```python
from build123d import *

# Parameters (mm, degrees)
F0_R     = 15
F0_R_2   = 13
F1_DEPTH = 2
F2_DEPTH = 20
F3_R     = 5
F4_SIZE  = 1.4
F5_R     = 1.4


with BuildPart() as f1:
    # F0 (on Top) → F1 (new body)
    with BuildSketch(Plane.XY):
        Circle(F0_R)
        Circle(F0_R_2, mode=Mode.SUBTRACT)
        Circle(F0_R_2)
    extrude(amount=F1_DEPTH)

    # F0 (on Top) → F2 (join)
    with BuildSketch(Plane.XY):
        Circle(F0_R)
        Circle(F0_R_2, mode=Mode.SUBTRACT)
    extrude(amount=F2_DEPTH)

    # F3
    f3_edges = [f1.edges().sort_by_distance(p)[0] for p in [
        (-13, 0, 2),
    ]]
    fillet(f3_edges, radius=F3_R)

    # F4
    f4_edges = [f1.edges().sort_by_distance(p)[0] for p in [
        (-13, 0, 20),
    ]]
    chamfer(f4_edges, length=F4_SIZE)

    # F5
    f5_edges = [f1.edges().sort_by_distance(p)[0] for p in [
        (-15, 0, 0),
    ]]
    fillet(f5_edges, radius=F5_R)


solid = f1.part
```
Geometry: final body of the model. Coordinates: model frame, mm. A direction names the side the tool comes from. Coordinates: 2 decimals unless noted, no trailing zeros. Loops run counter-clockwise (first coordinate to the right, second up) from the corner with the lowest first, then second, coordinate; pieces in that order, holes last. Notation, with made-up numbers: (10, 53) -> (35, 53) arc R21 cw to (35, 74) -> close; hole circle Ø7 at (35, -23.75). An arc over 180 degrees is marked (long way). Use a Markdown table: item, result. Add a question column.
(1) Section query A-A, the plane y = 0. Return loops of the section in (x, z).
(2) Mould query, pull axis Y, two halves, no side actions, for faces 3 (the cylindrical face through (-14.985, 0.66, 10.57)), 4 (the cylindrical face through (-10.316, -7.91, 12.719)), 5 (the flat face through (0, 0, 0)). Classes: pulls with the +Y half, pulls with the -Y half, needs draft (parallel to the pull), parting line crosses it, or undercut.
(3) Pin query (flat end, axial travel): pin 1 Ø12 at (x, y) = (-4, 3) entering from +Z; pin 2 Ø2 at (x, y) = (-6.5, 7.5) entering from +Z; pin 3 Ø1.5 at (x, z) = (7.5, 13.5) entering from +Y. Return the tip coordinate at first contact, or that it passes through.
(4) Access query for faces 1 (the flat face through (-7.8, 12.3, 20)), 2 (the flat face through (0, 0, 2)). Directions: +Z, -Z, +X, -X, +Y, -Y. A direction counts if a zero-diameter tool reaches every point of the face in a straight line with its end or side. Return the directions, or none.
(5) Section query C-C, the plane z = 12. Return loops of the section in (x, y), plus the area to 3 significant figures.
(6) Line query: line 1 along Y through (x, z) = (0, 10.75); line 2 along Z through (x, y) = (-5.25, -1.5); line 3 along X through (y, z) = (-6.5, 5.5). Output: solid intervals per line, ascending.
Answer:
| question | item | result |
|---|---|---|
| 1 | outline | (-15, 1.4) arc R1.4 ccw to (-13.6, 0) -> (13.6, 0) arc R1.4 ccw to (15, 1.4) -> (15, 20) -> (14.4, 20) -> (13, 18.6) -> (13, 7) arc R5 cw to (8, 2) -> (-8, 2) arc R5 cw to (-13, 7) -> (-13, 18.6) -> (-14.4, 20) -> (-15, 20) -> close |
| 2 | face 3 | parting line crosses it |
| 2 | face 4 | undercut |
| 2 | face 5 | needs draft |
| 3 | pin 1 | stops at z = 3 |
| 3 | pin 2 | stops at z = 2.94 |
| 3 | pin 3 | stops at y = 13.4 |
| 4 | face 1 | +Z, +X, -X, +Y, -Y |
| 4 | face 2 | +Z |
| 5 | outline | circle Ø30 at (0, 0); hole circle Ø26 at (0, 0) |
| 5 | area | 176 mm^2 |
| 6 | line 1 | y = -15 to -13, 13 to 15 |
| 6 | line 2 | z = 0 to 2 |
| 6 | line 3 | x = -13.52 to -10.99, 10.99 to 13.52 |
